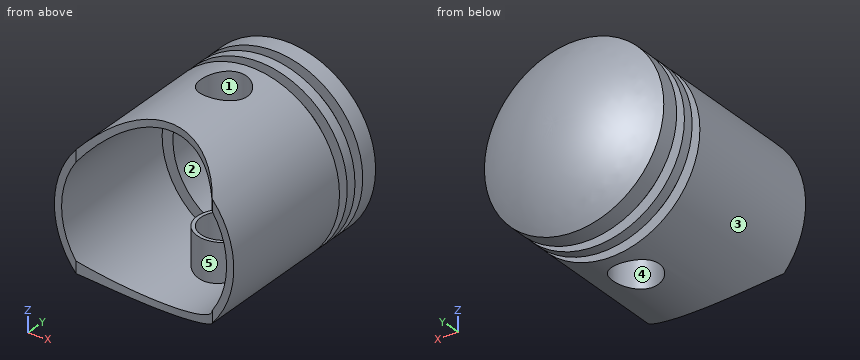
from build123d import *

# Parameters (mm, degrees)
SKETCH2_R               = 6.5
CUT_EXTRUDE2_DEPTH      = 26.0000001
CUT_EXTRUDE2_DEPTH_BACK = 26.0000001
BOSS_EXTRUDE1_START     = 12
SKETCH3_R               = 7.5
SKETCH3_R_2             = 6.5
BOSS_EXTRUDE1_DEPTH     = 11


with BuildPart() as part:
    # Sketch1 → Revolve9 (revolve)
    with BuildSketch(Plane.XY):
        with BuildLine():
            Line((-23, -31.5), (-23, 7.5))
            Line((-23, 7.5), (-20, 7.5))
            Line((-20, 7.5), (-20, 20.5))
            Line((-20, 20.5), (-23, 20.5))
            Line((-23, 20.5), (-23, 22.484511145))
            ThreePointArc((-23, 22.484511145), (-12.093024708, 27.851979987), (-0.04919363, 29.500605095))
            Line((-0.04919363, 29.500605095), (0, 29.500605095))
            Line((0, 29.500605095), (0, 31.5))
            ThreePointArc((0, 31.5), (-13.174901691, 29.609067785), (-25, 23.5))
            Line((-25, 23.5), (-25, 18.5))
            Line((-25, 18.5), (-22, 18.5))
            Line((-22, 18.5), (-22, 15.5))
            Line((-22, 15.5), (-25, 15.5))
            Line((-25, 15.5), (-25, 12.5))
            Line((-25, 12.5), (-22, 12.5))
            Line((-22, 12.5), (-22, 9.5))
            Line((-22, 9.5), (-25, 9.5))
            Line((-25, 9.5), (-25, -31.5))
            Line((-25, -31.5), (-23, -31.5))
        make_face()
    revolve(axis=Axis((0, -31.5, 0), (0, 1, 0)))

    # Sketch2 → Cut-Extrude2 (cut, two sides)
    with BuildSketch(Plane.XY) as cut_extrude2_sk:
        with Locations((0, -0.5)):
            Circle(SKETCH2_R)
        with BuildLine():
            Line((-19, -31.5), (19, -31.5))
            ThreePointArc((19, -31.5), (0, -21.5), (-19, -31.5))
        make_face()
    extrude(amount=CUT_EXTRUDE2_DEPTH, mode=Mode.SUBTRACT)
    extrude(cut_extrude2_sk.sketch, amount=-CUT_EXTRUDE2_DEPTH_BACK, mode=Mode.SUBTRACT)

    # Sketch3 → Boss-Extrude1 (add)
    with BuildSketch(Plane.XY.offset(BOSS_EXTRUDE1_START)):
        with Locations((0, -0.5)):
            Circle(SKETCH3_R)
        with Locations((0, -0.5)):
            Circle(SKETCH3_R_2, mode=Mode.SUBTRACT)
    boss_extrude1 = extrude(amount=BOSS_EXTRUDE1_DEPTH)

    # Mirror1: Boss-Extrude1 across plane
    add(boss_extrude1.mirror(Plane.XY))


solid = part.part
Work out the finished part from the listing and answer in its coordinate system (mm). Face numbers are marked on the shaded views. A direction names the side the tool comes from. Coordinates: 2 decimals unless noted, no trailing zeros. Write each loop counter-clockwise with the first axis right and the second up, starting at its lowest first coordinate (ties: lowest second). Pieces come first, ordered by that corner, then holes. Notation, with made-up numbers: M 67,19 L 74,19 A22 cw 74,25 Z; hole C -30.75,58.5 d4. An arc over 180 degrees is marked long. Answer as CSV lines item,"result". Start each with the question number.
Item 1: Flat-ended cylindrical pins translate along their axes: P1, Ø10.5, axis at x = 0, y = -0.5, coming from the -Z side; P2, Ø14, axis at x = 4, z = -11, coming from the +Y side; P3, Ø3, axis at y = -21, z = 12, coming from the -X side; P4, Ø10, axis at y = -18, z = 8, coming from the -X side. Find the tip coordinate at first contact, or state that the pin passes through.
Item 2: Determine the mould class of the marked faces 3, 4 and 5 for opening direction Z: released by +Z, released by -Z, zero draft, split by the parting line, or undercut.
Item 3: Section A-A on y = -0.5 is taken. Write down the section's boundary in (x, z), and give its area (3 significant figures).
Item 4: Consider L1, parallel to X at y = -2, z = -18; L2, parallel to Z at x = 0, y = -10.5; L3, parallel to Z at x = 0.5, y = 17.5. Determine where each line is inside the solid, lowest interval first.
Item 5: A tool of negligible diameter and unlimited length cuts with its end or side. For the marked faces 1 and 2, from which of +Z, -Z, +X, -X, +Y, -Y can it reach the whole face along a straight path? Write none if from no direction.
Item 6: Section B-B on z = 17.5 is taken. Give the number of separate pieces and of enclosed holes in the cut face, and give its area (3 significant figures).
Checks:
1,P1,"passes through"
1,P2,"stops at y = 31.34"
1,P3,"stops at x = -22.69"
1,P4,"stops at x = -24.82"
2,face 3,"split by the parting line"
2,face 4,"zero draft"
2,face 5,"undercut"
3,outline,"M -7.5,-21.74 A23 cw -7.5,21.74 L -7.5,12 L -6.5,12 L -6.5,24.14 A25 ccw -6.5,-24.14 L -6.5,-12 L -7.5,-12 Z; M 6.5,-24.14 A25 ccw 6.5,24.14 L 6.5,12 L 7.5,12 L 7.5,21.74 A23 cw 7.5,-21.74 L 7.5,-12 L 6.5,-12 Z"
3,area,"289 mm²"
4,L1,"x = -17.35 to -14.32, -7.35 to -6.32, 6.32 to 7.35, 14.32 to 17.35"
4,L2,"z = -25 to -23, 23 to 25"
4,L3,"z = -21.99 to -19.99, 19.99 to 21.99"
5,face 1,"+Z, -Z"
5,face 2,"none"
6,separate pieces,"2"
6,enclosed holes,"1"
6,area,"502 mm²"
